```python
from build123d import *

# Parameters (mm, degrees)
CROQUIS2_W              = 70
CROQUIS2_H              = 40
SALIENTE_EXTRUIR1_DEPTH = 45
CROQUIS3_W              = 40.5
CROQUIS3_H              = 20
CORTAR_EXTRUIR1_DEPTH   = 39
CROQUIS4_W              = 7
CROQUIS4_H              = 20
CORTAR_EXTRUIR2_DEPTH   = 12
CROQUIS5_W              = 20
CROQUIS5_H              = 20
CORTAR_EXTRUIR4_DEPTH   = 7
CROQUIS6_R              = 7.5
SALIENTE_EXTRUIR3_DEPTH = 30
CROQUIS8_R              = 7.5
SALIENTE_EXTRUIR4_DEPTH = 30
CROQUIS9_W              = 30
CROQUIS9_H              = 40
SALIENTE_EXTRUIR5_DEPTH = 10
CROQUIS10_R             = 7.5
SALIENTE_EXTRUIR6_DEPTH = 54
REDONDEO1_R             = 5
CROQUIS11_W             = 42.231434226
CROQUIS11_H             = 4
CROQUIS11_W_2           = 30
CORTAR_EXTRUIR7_DEPTH   = 60
CROQUIS12_R             = 7.5
SALIENTE_EXTRUIR7_DEPTH = 100
CROQUIS13_W             = 75.549853641
CROQUIS13_H             = 40.129267471
CORTAR_EXTRUIR8_DEPTH   = 100


with BuildPart() as part:
    # Croquis2 → Saliente-Extruir1 (new body)
    with BuildSketch(Plane.XY):
        with Locations((35, 20)):
            Rectangle(CROQUIS2_W, CROQUIS2_H)
    extrude(amount=SALIENTE_EXTRUIR1_DEPTH)

    # Croquis3 → Cortar-Extruir1 (cut)
    with BuildSketch(Plane(origin=(0, 0, 0), x_dir=(-1, 0, 0), z_dir=(0, 0, -1))):
        with Locations((-27.25, 20)):
            Rectangle(CROQUIS3_W, CROQUIS3_H)
    extrude(amount=-CORTAR_EXTRUIR1_DEPTH, mode=Mode.SUBTRACT)

    # Croquis4 → Cortar-Extruir2 (cut)
    with BuildSketch(Plane(origin=(0, 0, 0), x_dir=(-1, 0, 0), z_dir=(0, 0, -1))):
        with Locations((-3.5, 20)):
            Rectangle(CROQUIS4_W, CROQUIS4_H)
        with Locations((-51, 20)):
            Rectangle(CROQUIS4_W, CROQUIS4_H)
    extrude(amount=-CORTAR_EXTRUIR2_DEPTH, mode=Mode.SUBTRACT)

    # Croquis5 → Cortar-Extruir4 (cut)
    with BuildSketch(Plane.ZY):
        with Locations((35, 20)):
            Rectangle(CROQUIS5_W, CROQUIS5_H)
    extrude(amount=-CORTAR_EXTRUIR4_DEPTH, mode=Mode.SUBTRACT)

    # Croquis6 → Saliente-Extruir3 (add)
    with BuildSketch(Plane(origin=(0, 40, 0), x_dir=(1, 0, 0), z_dir=(0, 1, 0))):
        with Locations((52.5, -22.5)):
            Circle(CROQUIS6_R)
    extrude(amount=SALIENTE_EXTRUIR3_DEPTH)

    # Croquis8 → Saliente-Extruir4 (add)
    with BuildSketch(Plane.XZ):
        with Locations((52.5, 22.5)):
            Circle(CROQUIS8_R)
    extrude(amount=SALIENTE_EXTRUIR4_DEPTH)

    # Croquis9 → Saliente-Extruir5 (add)
    with BuildSketch(Plane(origin=(0, 0, 0), x_dir=(-1, 0, 0), z_dir=(0, 0, -1))):
        with Locations((-15, 20)):
            Rectangle(CROQUIS9_W, CROQUIS9_H)
    extrude(amount=SALIENTE_EXTRUIR5_DEPTH)

    # Croquis10 → Saliente-Extruir6 (add)
    with BuildSketch(Plane(origin=(0, 0, -10), x_dir=(-1, 0, 0), z_dir=(0, 0, -1))):
        with Locations((-15, 20)):
            Circle(CROQUIS10_R)
    extrude(amount=SALIENTE_EXTRUIR6_DEPTH)

    # Redondeo1
    redondeo1_edges = [part.edges().sort_by_distance(p)[0] for p in [
        (70, 20, 0),
    ]]
    fillet(redondeo1_edges, radius=REDONDEO1_R)

    # Croquis11 → Cortar-Extruir7 (cut)
    with BuildSketch(Plane(origin=(0, 0, -10), x_dir=(-1, 0, 0), z_dir=(0, 0, -1))):
        with Locations((-51.115717113, 2)):
            Rectangle(CROQUIS11_W, CROQUIS11_H)
        with Locations((-51.115717113, 38)):
            Rectangle(CROQUIS11_W, CROQUIS11_H)
        with Locations((-15, 38)):
            Rectangle(CROQUIS11_W_2, CROQUIS11_H)
        with Locations((-15, 2)):
            Rectangle(CROQUIS11_W_2, CROQUIS11_H)
    extrude(amount=-CORTAR_EXTRUIR7_DEPTH, mode=Mode.SUBTRACT)

    # Croquis12 → Saliente-Extruir7 (add)
    with BuildSketch(Plane(origin=(0, 70, 0), x_dir=(1, 0, 0), z_dir=(0, 1, 0))):
        with Locations((52.5, -22.5)):
            Circle(CROQUIS12_R)
    extrude(amount=-SALIENTE_EXTRUIR7_DEPTH)

    # Croquis13 → Cortar-Extruir8 (cut)
    with BuildSketch(Plane(origin=(0, 0, -10), x_dir=(-1, 0, 0), z_dir=(0, 0, -1))):
        with Locations((-37.77492682, -26.064633736)):
            Rectangle(CROQUIS13_W, CROQUIS13_H)
        with Locations((-37.77492682, 66.064633735)):
            Rectangle(CROQUIS13_W, CROQUIS13_H)
    extrude(amount=-CORTAR_EXTRUIR8_DEPTH, mode=Mode.SUBTRACT)


solid = part.part
```
Part model, mm, in its own coordinate system. A direction names the side the tool comes from. Round coordinates to 2 decimals unless told otherwise and drop trailing zeros. Write each loop counter-clockwise with the first axis right and the second up, starting at its lowest first coordinate (ties: lowest second). Pieces come first, ordered by that corner, then holes. Notation, with made-up numbers: M 6.5,-21.5 L 14.5,-21.5 A10 cw 14.5,-17.5 Z; hole C 2,40 d2. An arc over 180 degrees is marked long. One line per question, with ' | ' between items.
(1) Saw through at C-C on z = 22.5. Write the cut outline in (x, y).
Answer key:
outline: M 0,4 L 45,4 L 45,-6 L 60,-6 L 60,4 L 70,4 L 70,36 L 60,36 L 60,46 L 45,46 L 45,36 L 0,36 Z; hole M 7,10 L 45,10 L 45,30 L 7,30 Z
(2) Saw through at B-B on y = 20. Write the cut outline in (x, z).
Answer key:
outline: M 0,-10 L 7.5,-10 L 7.5,-64 L 22.5,-64 L 22.5,-10 L 30,-10 L 30,0 L 0,0 Z; M 0,12 L 7,12 L 7,25 L 0,25 Z; M 7,39 L 47.5,39 L 47.5,28.09 A7.5 ccw 47.5,16.91 L 47.5,12 L 54.5,12 L 54.5,0 L 65,0 A5 ccw 70,5 L 70,45 L 7,45 Z
(3) Probe line 1 along Y through (x, z) = (37, 33); line 2 along Z through (x, y) = (26, 29.5); line 3 along Z through (x, y) = (59, 15). List the from-to ranges inside material, lowest first.
Answer key:
line 1: y = 4 to 10, 30 to 36 | line 2: z = -10 to 0, 39 to 45 | line 3: z = 0 to 45
(4) Pin check, flat tips, straight feed: pin 1 (11 mm diameter, centred on y = 16.5, z = -5, fed in from +X); pin 2 (5 mm diameter, centred on x = 9, z = 31, fed in from -Y); pin 3 (12 mm diameter, centred on y = 8.5, z = -28.5, fed in from -X); pin 4 (12 mm diameter, centred on y = 36, z = -25, fed in from +X). Stop position of each tip, or through.
Answer key:
pin 1: stops at x = 67.18 | pin 2: stops at y = 4 | pin 3: stops at x = 9.9 | pin 4: passes through
(5) Saw through at D-D on y = 32.5. Write the cut outline in (x, z).
Answer key:
outline: M 0,-10 L 30,-10 L 30,0 L 65,0 A5 ccw 70,5 L 70,45 L 0,45 Z
(6) Saw through at A-A on x = 21. Write the cut outline in (y, z).
Answer key:
outline: M 4,-10 L 15.5,-10 L 15.5,-64 L 24.5,-64 L 24.5,-10 L 36,-10 L 36,45 L 4,45 Z; hole M 10,0 L 30,0 L 30,39 L 10,39 Z
(7) 3-axis set-ups, long thin cutter, end or side, ignore diameter. For faces 5 (the face through (3, 20, 25)), 6 (the face through (7, 20, 18)), 7 (the face through (22, 24, -10)), 8 (the face through (54.5, 20, 6)), 9 (the face through (15, 20, 0)): which of +Z, -Z, +X, -X, +Y, -Y reach the whole face in a straight line?
Answer key:
face 5: +Z, -X | face 6: none | face 7: -Z | face 8: -Z, -X | face 9: -X
(8) Two-plate mould, pull along Z, no slides. Class faces 1 (the face through (28, 30, 17)), 2 (the face through (53, 46, 22)), 3 (the face through (28, 10, 17)), 4 (the face through (51, 20, 12)): released by +Z, released by -Z, zero draft, split by the parting line, or undercut.
Answer key:
face 1: undercut | face 2: zero draft | face 3: undercut | face 4: released by -Z
